Here's how the part is built. I have some questions about the finished solid (model axes, mm). A direction names the side the tool comes from. Give positions to 0.01 mm unless a question says otherwise; leave off trailing zeros. Order: outer loops, then holes, each group sorted by start corner. A loop starts at its lowest first (then second) coordinate and runs counter-clockwise, first axis right, second up. Notation, with made-up numbers: (-10.75, 19) -> (29.25, 19) arc R22 ccw to (29.25, 56) -> close; hole circle Ø3 at (-24.5, -22.5). An arc over 180 degrees is marked (long way). Write each question's results on one line, items separated by ' | '. Start each with the question number.
Q1. Imagine slicing it at B-B, the plane x = -53. Please give me the cut outline in (y, z) (3 decimals), then the cut area to 3 significant figures.
Q2. I'm going to push flat-ended pins straight in: pin 1 (6 mm diameter, centred on x = -42.5, y = 39, fed in from +Z); pin 2 (10 mm diameter, centred on y = 20, z = -48, fed in from -X); pin 3 (8 mm diameter, centred on x = -10.5, z = -4.5, fed in from -Y) (3 decimals). Where does each tip first touch, or does it pass through?
Q3. I need wall thicknesses on line 1 along X through (y, z) = (37, -0.5); line 2 along X through (y, z) = (22.5, 19); line 3 along Y through (x, z) = (38, 36.5) (3 decimals). Which ranges of each line are inside material? Lowest first, please. Write a range as [from, to].
Q4. For faces 1 (the face through (-6, 0, -5)), 2 (the face through (-6.35, 23, 1)), which set-ups out of +Z, -Z, +X, -X, +Y, -Y let a thin tool reach every point of the face, with its end or its side?
Q5. Imagine slicing it at A-A, the plane y = 19.5. Please give me the cut outline in (x, z) (3 decimals).
Q6. Thinking about a two-plate mould opening in X: for faces 3 (the face through (63.487, 23.479, -1.307)), 4 (the face through (-1, 57.15, 1)), which applies, pulls with the +X half, pulls with the -X half, needs draft (parallel to the pull), parting line crosses it, or undercut?
Q7. Imagine slicing it at C-C, the plane z = -50.5. Please give me the cut outline in (x, y) (3 decimals).
Q8. Imagine slicing it at D-D, the plane x = -23.5. Please give me the cut outline in (y, z) (3 decimals), then the cut area to 3 significant figures.
```python
from build123d import *

# Parameters (mm, degrees)
F2_DEPTH = 57.15
F1_R     = 63.5
F3_DEPTH = 47.625
F4_DEPTH = 47.625


with BuildPart() as f2:
    # F0 (on Front) → F2 (new body)
    with BuildSketch(Plane.XZ):
        with BuildLine():
            Line((-6.35, 0), (-6.35, 72.7483891574))
            ThreePointArc((-6.35, 72.7483891574), (-73.025, 0), (-6.35, -72.7483891574))
            Line((-6.35, -72.7483891574), (-6.35, 0))
        make_face()
        with BuildLine():
            ThreePointArc((6.35, -72.7483891574), (53.8347442411, -49.3403581006), (73.025, 0))
            ThreePointArc((73.025, 0), (53.8347442411, 49.3403581006), (6.35, 72.7483891574))
            Line((6.35, 72.7483891574), (6.35, 0))
            Line((6.35, 0), (6.35, -72.7483891574))
        make_face()
        with BuildLine():
            Line((6.35, 0), (6.35, 72.7483891574))
            ThreePointArc((6.35, 72.7483891574), (0, 73.025), (-6.35, 72.7483891574))
            Line((-6.35, 72.7483891574), (-6.35, 0))
            Line((-6.35, 0), (0, 0))
            Line((0, 0), (6.35, 0))
        make_face()
        with BuildLine():
            ThreePointArc((-6.35, -72.7483891574), (0, -73.025), (6.35, -72.7483891574))
            Line((6.35, -72.7483891574), (6.35, 0))
            Line((6.35, 0), (0, 0))
            Line((0, 0), (-6.35, 0))
            Line((-6.35, 0), (-6.35, -72.7483891574))
        make_face()
    extrude(amount=-F2_DEPTH)

    # F1 (on Front) → F3 (cut)
    with BuildSketch(Plane.XZ):
        Circle(F1_R)
    extrude(amount=-F3_DEPTH, mode=Mode.SUBTRACT)

    # F0 (on Front) → F4 (join)
    with BuildSketch(Plane.XZ):
        with BuildLine():
            ThreePointArc((-6.35, -72.7483891574), (0, -73.025), (6.35, -72.7483891574))
            Line((6.35, -72.7483891574), (6.35, 0))
            Line((6.35, 0), (0, 0))
            Line((0, 0), (-6.35, 0))
            Line((-6.35, 0), (-6.35, -72.7483891574))
        make_face()
        with BuildLine():
            Line((6.35, 0), (6.35, 72.7483891574))
            ThreePointArc((6.35, 72.7483891574), (0, 73.025), (-6.35, 72.7483891574))
            Line((-6.35, 72.7483891574), (-6.35, 0))
            Line((-6.35, 0), (0, 0))
            Line((0, 0), (6.35, 0))
        make_face()
    extrude(amount=-F4_DEPTH)


solid = f2.part
```
Geometry check:
1) outline: (0, -50.236) -> (57.15, -50.236) -> (57.15, 50.236) -> (0, 50.236) -> (0, 34.975) -> (47.625, 34.975) -> (47.625, -34.975) -> (0, -34.975) -> close | area: 2,410 mm²
2) pin 1: z = 61.42 | pin 2: x = -59.02 | pin 3: y = 47.625
3) line 1: [-73.02, -63.5], [-6.35, 6.35], [63.5, 73.02] | line 2: [-70.51, -60.59], [-6.35, 6.35], [60.59, 70.51] | line 3: [47.625, 57.15]
4) face 1: +Z, -Z, +X, -X, -Y | face 2: -Y
5) outline: circle Ø146.05 at (0, 0); hole (-6.35, -63.182) -> (-6.35, 63.182) arc R63.5 ccw to start; hole (6.35, -63.182) arc R63.5 ccw to (6.35, 63.182) -> close
6) face 3: undercut | face 4: needs draft
7) outline: (-52.748, 0) -> (-38.497, 0) -> (-38.497, 47.625) -> (-6.35, 47.625) -> (-6.35, 0) -> (6.35, 0) -> (6.35, 47.625) -> (38.497, 47.625) -> (38.497, 0) -> (52.748, 0) -> (52.748, 57.15) -> (-52.748, 57.15) -> close
8) outline: (0, -69.14) -> (57.15, -69.14) -> (57.15, 69.14) -> (0, 69.14) -> (0, 58.992) -> (47.625, 58.992) -> (47.625, -58.992) -> (0, -58.992) -> close | area: 2,280 mm²
